Input: part model. Units: mm. Frame: model coordinates. Coordinates: 2 decimals unless noted, no trailing zeros. Write each loop counter-clockwise with the first axis right and the second up, starting at its lowest first coordinate (ties: lowest second). Pieces come first, ordered by that corner, then holes. Notation, with made-up numbers: (19, 53.25) - (31, 53.25) arc R24 cw to (31, 64.25) - close; hole circle Ø9 at (38, 52.5). An arc over 180 degrees is marked (long way). Use a Markdown table: item, result. Add a question column.
Q1. Section query B-B (z = 0). Return the cut outline in (x, y).
Q2. Section query C-C (y = 0.85). Return the cut outline in (x, z) (3 decimals), then the cut area to 3 significant figures.
Q3. Section query A-A (x = 0). Return the cut outline in (y, z).
Q4. Material intervals for probe 1 along X at (y, z) = (2, 0); probe 2 along Z at (x, y) = (-12, 2.2); probe 3 along X at (y, z) = (1.9, 21.5), sorted ascending. Write a range as from..to.
Q5. Section query D-D (x = 25.15). Return the cut outline in (y, z).
from build123d import *

# Parameters (mm, degrees)
SKETCH1_R           = 30
SKETCH1_R_2         = 1.5
SKETCH1_R_3         = 14
BOSS_EXTRUDE1_DEPTH = 3


with BuildPart() as part:
    # Sketch1 → Boss-Extrude1 (new body)
    with BuildSketch(Plane(origin=(0, 0, 0), x_dir=(1, 0, 0), z_dir=(0, 1, 0))):
        Circle(SKETCH1_R)
        with Locations((-25.15, 0)):
            Circle(SKETCH1_R_2, mode=Mode.SUBTRACT)
        Circle(SKETCH1_R_3, mode=Mode.SUBTRACT)
        with Locations((-12.575, 21.780538905)):
            Circle(SKETCH1_R_2, mode=Mode.SUBTRACT)
        with Locations((12.575, 21.780538905)):
            Circle(SKETCH1_R_2, mode=Mode.SUBTRACT)
        with Locations((25.15, 0)):
            Circle(SKETCH1_R_2, mode=Mode.SUBTRACT)
        with Locations((12.575, -21.780538905)):
            Circle(SKETCH1_R_2, mode=Mode.SUBTRACT)
        with Locations((-12.575, -21.780538905)):
            Circle(SKETCH1_R_2, mode=Mode.SUBTRACT)
    extrude(amount=BOSS_EXTRUDE1_DEPTH)


solid = part.part
Values follow:
| question | item | result |
|---|---|---|
| 1 | outline | (-30, 0) - (-26.65, 0) - (-26.65, 3) - (-30, 3) - close; (-23.65, 0) - (-14, 0) - (-14, 3) - (-23.65, 3) - close; (14, 0) - (23.65, 0) - (23.65, 3) - (14, 3) - close; (26.65, 0) - (30, 0) - (30, 3) - (26.65, 3) - close |
| 2 | outline | circle Ø60 at (0, 0); hole circle Ø3 at (-25.15, 0); hole circle Ø3 at (-12.575, -21.781); hole circle Ø3 at (-12.575, 21.781); hole circle Ø28 at (0, 0); hole circle Ø3 at (12.575, -21.781); hole circle Ø3 at (12.575, 21.781); hole circle Ø3 at (25.15, 0) |
| 2 | area | 2,170 mm2 |
| 3 | outline | (0, -30) - (3, -30) - (3, -14) - (0, -14) - close; (0, 14) - (3, 14) - (3, 30) - (0, 30) - close |
| 4 | probe 1 | -30..-26.65, -23.65..-14, 14..23.65, 26.65..30 |
| 4 | probe 2 | -27.5..-23.17, -20.4..-7.21, 7.21..20.4, 23.17..27.5 |
| 4 | probe 3 | -20.92..-14.05, -11.1..11.1, 14.05..20.92 |
| 5 | outline | (0, -16.35) - (3, -16.35) - (3, -1.5) - (0, -1.5) - close; (0, 1.5) - (3, 1.5) - (3, 16.35) - (0, 16.35) - close |
